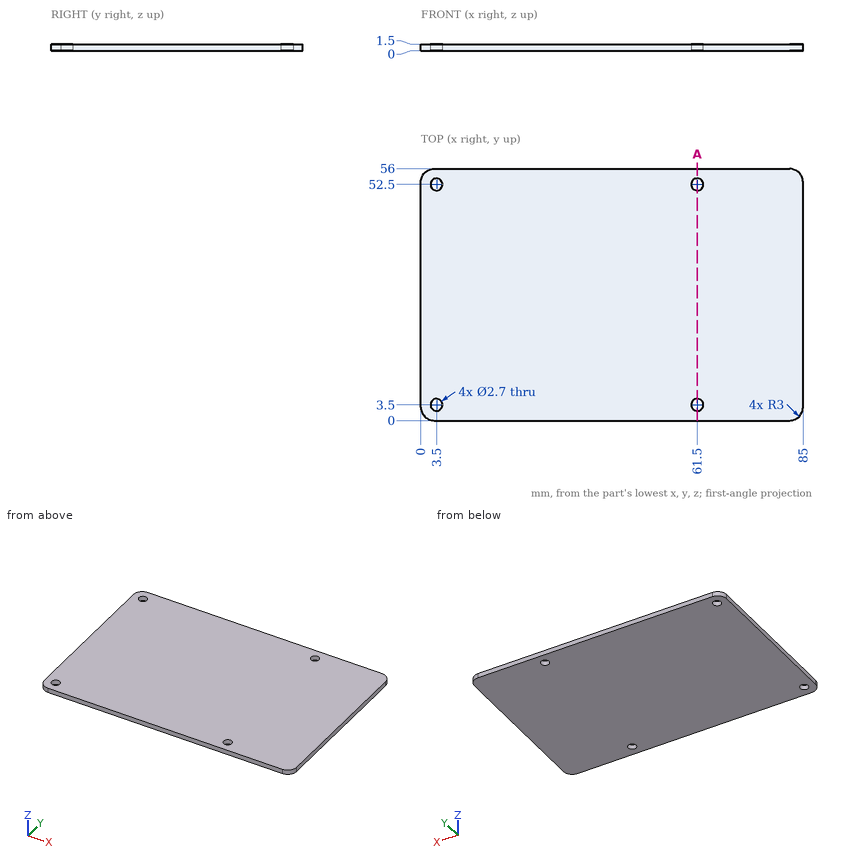
The figure shows three views and two pictorial views of one solid part (mm, origin at its lowest corner). Answer the questions. Round coordinates to 2 decimals unless told otherwise and drop trailing zeros. Order: outer loops, then holes, each group sorted by start corner. A loop starts at its lowest first (then second) coordinate and runs counter-clockwise, first axis right, second up. Notation, with made-up numbers: M 81.5,71.5 L 113.5,71.5 A4 ccw 113.5,78.5 Z; hole C 76.5,-1.75 d6. An arc over 180 degrees is marked long. Put each result on its own line as item: value. Start each with the question number.
Q1. Flat-ended cylindrical pins translate along their axes: pin 1 (3 mm diameter, centred on x = 61.5, y = 52.5, fed in from -Z); pin 2 (1.6 mm diameter, centred on x = 3.5, y = 3.5, fed in from -Z). Find the tip coordinate at first contact, or state that the pin passes through.
Q2. Section A-A, the plane x = 61.5 is taken. Write down the section's boundary in (y, z), and give its area (3 significant figures).
Q3. Straight lines are drawn through the part: L1, parallel to Y at x = 61.5, z = 0.9; L2, parallel to X at y = 53.5, z = 1.25. For each, find the intervals that lie inside material, in ascending order. Write a range as [from, to].
Findings below:
1. pin 1: stops at z = 0
1. pin 2: passes through
2. outline: M 0,0 L 2.15,0 L 2.15,1.5 L 0,1.5 Z; M 4.85,0 L 51.15,0 L 51.15,1.5 L 4.85,1.5 Z; M 53.85,0 L 56,0 L 56,1.5 L 53.85,1.5 Z
2. area: 75.9 mm^2
3. L1: y = [0, 2.15], [4.85, 51.15], [53.85, 56]
3. L2: x = [0.04, 2.59], [4.41, 60.59], [62.41, 84.96]
